Here's the drawing with two shaded views (mm, measured from the low corner). I have some questions. Coordinates: 2 decimals unless noted, no trailing zeros. Loops run counter-clockwise (first coordinate to the right, second up) from the corner with the lowest first, then second, coordinate; pieces in that order, holes last. Notation, with made-up numbers: (-9, 51.5) - (-1, 51.5) arc R26 ccw to (-1, 76.5) - close; hole circle Ø7 at (58, -17.75). An arc over 180 degrees is marked (long way). Use a Markdown table: item, result.
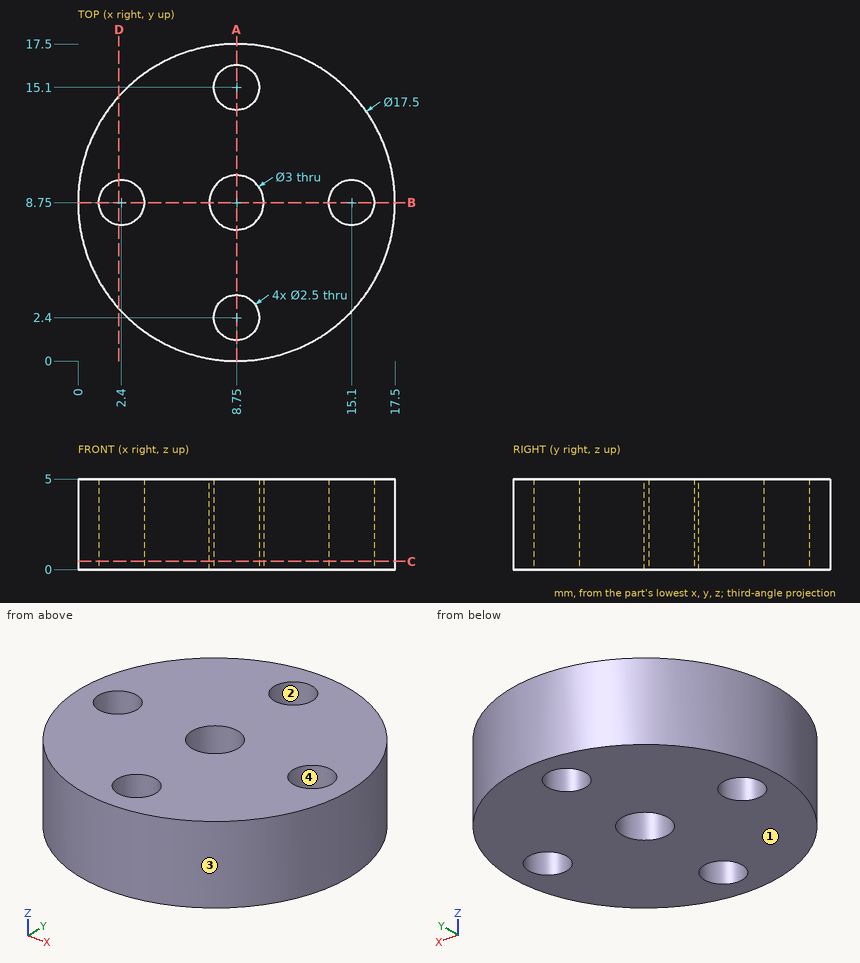
Q1. If we mould it in two halves opening along X, with no side actions, what happens to the marked faces 1, 2, 3 and 4? For each: pulls with the +X half, pulls with the -X half, needs draft (parallel to the pull), parting line crosses it, or undercut.
Check values:
| item | result |
|---|---|
| face 1 | needs draft |
| face 2 | undercut |
| face 3 | parting line crosses it |
| face 4 | undercut |
Q2. I want a section at D-D, the plane x = 2.25. Write out the boundary of the cut face in (y, z).
Check values:
| item | result |
|---|---|
| outline | (2.89, 0) - (7.51, 0) - (7.51, 5) - (2.89, 5) - close; (9.99, 0) - (14.61, 0) - (14.61, 5) - (9.99, 5) - close |
Q3. Please list where these lines run through material, in increasing order: L1, parallel to Y at x = 8.75, z = 2.9; L2, parallel to X at y = 9.25, z = 2.75; L3, parallel to Y at x = 15.1, z = 1.55. Write a range as from..to.
Check values:
| item | result |
|---|---|
| L1 | 0..1.15, 3.65..7.25, 10.25..13.85, 16.35..17.5 |
| L2 | 0.01..1.25, 3.55..7.34, 10.16..13.95, 16.25..17.49 |
| L3 | 2.73..7.5, 10..14.77 |
Q4. I want a section at C-C, the plane z = 0.45. Write out the boundary of the cut face in (x, y), then the cut area to 3 significant figures.
Check values:
| item | result |
|---|---|
| outline | circle Ø17.5 at (8.75, 8.75); hole circle Ø2.5 at (2.4, 8.75); hole circle Ø3 at (8.75, 8.75); hole circle Ø2.5 at (8.75, 2.4); hole circle Ø2.5 at (8.75, 15.1); hole circle Ø2.5 at (15.1, 8.75) |
| area | 214 mm^2 |
Q5. I want a section at A-A, the plane x = 8.75. Write out the boundary of the cut face in (y, z), then the cut area to 3 significant figures.
Check values:
| item | result |
|---|---|
| outline | (0, 0) - (1.15, 0) - (1.15, 5) - (0, 5) - close; (3.65, 0) - (7.25, 0) - (7.25, 5) - (3.65, 5) - close; (10.25, 0) - (13.85, 0) - (13.85, 5) - (10.25, 5) - close; (16.35, 0) - (17.5, 0) - (17.5, 5) - (16.35, 5) - close |
| area | 47.5 mm^2 |
